Autodesk Inventor part; units mm, degrees
ref_plane "Work Plane1" through (0, 0, 13.5128) normal (0, 0, 1) x (1, 0, 0)
ref_plane "YZ Plane" through (0, 0, 0) normal (1, 0, 0) x (0, 1, 0)
ref_plane "XZ Plane" through (0, 0, 0) normal (0, 1, 0) x (-1, 0, 0)
sketch "Sketch1" plane through (0, 0, 0) normal (0, 0, 1) x (1, 0, 0)
  line L0 (-12.7, 5.08) -> (12.7, 5.08)
  line L1 (12.7, 5.08) -> (12.7, -5.08)
  line L2 (12.7, -5.08) -> (-12.7, -5.08)
  line L3 (-12.7, -5.08) -> (-12.7, 5.08)
  point P0 (0, 0)
  point P1 (0, 5.08)
  point P2 (-12.7, 0)
  dimension "d0" = 25.4
  dimension "d1" = 10.16
extrude "Extrusion1" add sketch "Sketch1" along normal blind 0.8128
ref_plane "Work Plane1" through (0, 0, 13.5128) normal (0, 0, 1) x (1, 0, 0)
sketch "Sketch2" plane through (0, 0, 13.5128) normal (0, 0, 1) x (1, 0, 0)
  line L0 (12.7, 5.08) -> (12.7, -5.08)
  line L1 (-12.7, 5.08) -> (12.7, 5.08)
  line L2 (-12.7, -5.08) -> (-12.7, 5.08)
  line L3 (12.7, -5.08) -> (-12.7, -5.08)
  line L4 (-3.3655, 3.556) -> (3.3655, 3.556)
  line L5 (-3.3655, -3.556) -> (3.3655, -3.556)
  line L6 (-4.953, 1.9685) -> (-4.953, -1.9685)
  line L7 (4.953, 1.9685) -> (4.953, -1.9685)
  arc A0 (-3.3655, 3.556) -> (-4.953, 1.9685) centre (-3.3655, 1.9685) ccw
  arc A1 (-4.953, -1.9685) -> (-3.3655, -3.556) centre (-3.3655, -1.9685) ccw
  arc A2 (3.3655, -3.556) -> (4.953, -1.9685) centre (3.3655, -1.9685) ccw
  arc A3 (4.953, 1.9685) -> (3.3655, 3.556) centre (3.3655, 1.9685) ccw
  point P0 (0, 0)
  point P1 (0, 3.556)
  point P2 (0, -3.556)
  point P3 (-4.953, 0)
  point P4 (4.953, 0)
  dimension "d5" = 6.731
  dimension "d6" = 6.731
  dimension "d7" = 3.937
  dimension "d8" = 3.937
  dimension "d9" = 4.953
  dimension "d10" = 4.953
  dimension "d11" = 3.556
  dimension "d12" = 3.556
  dimension "d13" = 1.5875
  dimension "d14" = 1.5875
  dimension "d15" = 1.5875
  dimension "d16" = 1.5875
extrude "Extrusion2" cut sketch "Sketch2" against normal blind 25.4 contours L4 A3 L7 A2 L5 A1 L6 A0
sketch "Sketch3" plane through (0, 0, 13.5128) normal (0, 0, 1) x (1, 0, 0)
  arc A0 (-3.3655, 3.556) -> (-4.953, 1.9685) centre (-3.3655, 1.9685) ccw
  line L0 (-3.3655, 3.556) -> (3.3655, 3.556)
  arc A1 (4.953, 1.9685) -> (3.3655, 3.556) centre (3.3655, 1.9685) ccw
  line L1 (4.953, 1.9685) -> (4.953, -1.9685)
  arc A2 (3.3655, -3.556) -> (4.953, -1.9685) centre (3.3655, -1.9685) ccw
  line L2 (3.3655, -3.556) -> (-3.3655, -3.556)
  arc A3 (-4.953, -1.9685) -> (-3.3655, -3.556) centre (-3.3655, -1.9685) ccw
  line L3 (-4.953, -1.9685) -> (-4.953, 1.9685)
  line L4 (12.7, 5.08) -> (12.7, -5.08)
  line L5 (-12.7, 5.08) -> (12.7, 5.08)
  line L6 (-12.7, -5.08) -> (-12.7, 5.08)
  line L7 (12.7, -5.08) -> (-12.7, -5.08)
  line L8 (-12.7, 1.5875) -> (-8.128, 1.5875)
  line L9 (-12.7, -1.5875) -> (-8.128, -1.5875)
  arc A4 (-8.128, -1.5875) -> (-8.128, 1.5875) centre (-8.128, 0) ccw
  point P0 (0, 0)
  dimension "d19" = 4.572
  dimension "d20" = 3.4925
  dimension "d21" = 4.572
  dimension "d22" = 3.175
  dimension "d24" = 1.5875
extrude "Extrusion3" cut sketch "Sketch3" against normal blind 25.4 contours L8 A4 L9 L6
mirror "Mirror1" about plane through (0, 0, 0) normal (1, 0, 0) of "Extrusion3"
properties part number "headplate_largerCenter"
CAD build for the part. Positions are in the model's coordinates, mm. A direction names the side the tool comes from. Round coordinates to 2 decimals unless told otherwise and drop trailing zeros. Loops run counter-clockwise (first coordinate to the right, second up) from the corner with the lowest first, then second, coordinate; pieces in that order, holes last. Notation, with made-up numbers: (37.25, 26.25) - (57.25, 26.25) arc R22 cw to (57.25, 59.25) - close; hole circle Ø11 at (-7, 62.25). An arc over 180 degrees is marked (long way). Return JSON: item names as keys, results as strings. Group by question number.
Q1. Band-saw the part on A-A on x = -3. Give the cut face in (y, z), plus the area to 3 significant figures.
Q2. Tool access for faces 5 (the face through (-10.4, -1.588, 0.4)), 6 (the face through (-12.7, -3.4, 0.4)), 7 (the face through (10.4, 1.588, 0.4)), 8 (the face through (4.5, 3.08, 0.41)), 9 (the face through (12.7, 3.4, 0.4)): list every direction of +Z, -Z, +X, -X, +Y, -Y with a clear straight run to the whole face (end or side of a thin tool).
Q3. Two-plate mould, pull along X, no slides. Class faces 1 (the face through (-4.48, 3.1, 0.41)), 2 (the face through (-10.4, 1.588, 0.4)), 3 (the face through (4.953, 0, 0.4)), 4 (the face through (-12.7, 3.3, 0.4)): +X half, -X half, draft (parallel to the pull), parting line (faces both ways), or undercut.
Q4. Drill centre lines: line 1 along X through (y, z) = (0, 0.75); line 2 along Y through (x, z) = (-9.25, 0.3); line 3 along X through (y, z) = (-3.25, 0.4). Where is each one in solid material? Low to high. Write a range as [from, to].
Q5. Band-saw the part on B-B on z = 0.25. Give the cut face in (x, y) (1 decimal), plus the area to 3 significant figures.
Q6. Band-saw the part on C-C on y = 0. Give the cut face in (x, z).
Solutions:
{
 "1": {"outline": "(-5.08, 0) - (-3.56, 0) - (-3.56, 0.81) - (-5.08, 0.81) - close; (3.56, 0) - (5.08, 0) - (5.08, 0.81) - (3.56, 0.81) - close", "area": "2.48 mm^2"},
 "2": {"face 5": "+Z, -Z, -X", "face 6": "+Z, -Z, -X, +Y, -Y", "face 7": "+Z, -Z, +X", "face 8": "+Z, -Z", "face 9": "+Z, -Z, +X, +Y, -Y"},
 "3": {"face 1": "undercut", "face 2": "draft", "face 3": "undercut", "face 4": "-X half"},
 "4": {"line 1": "x = [-6.54, -4.95], [4.95, 6.54]", "line 2": "y = [-5.08, -1.59], [1.59, 5.08]", "line 3": "x = [-12.7, -4.3], [4.3, 12.7]"},
 "5": {"outline": "(-12.7, -5.1) - (12.7, -5.1) - (12.7, -1.6) - (8.1, -1.6) arc R1.6 cw to (8.1, 1.6) - (12.7, 1.6) - (12.7, 5.1) - (-12.7, 5.1) - (-12.7, 1.6) - (-8.1, 1.6) arc R1.6 cw to (-8.1, -1.6) - (-12.7, -1.6) - close; hole (-5, -2) arc R1.6 ccw to (-3.4, -3.6) - (3.4, -3.6) arc R1.6 ccw to (5, -2) - (5, 2) arc R1.6 ccw to (3.4, 3.6) - (-3.4, 3.6) arc R1.6 ccw to (-5, 2) - close", "area": "153 mm^2"},
 "6": {"outline": "(-6.54, 0) - (-4.95, 0) - (-4.95, 0.81) - (-6.54, 0.81) - close; (4.95, 0) - (6.54, 0) - (6.54, 0.81) - (4.95, 0.81) - close"}
}
